The listing builds one solid part. Answer for the finished solid, in the listing's coordinates (mm). Coordinates: 2 decimals unless noted, no trailing zeros. Loops run counter-clockwise (first coordinate to the right, second up) from the corner with the lowest first, then second, coordinate; pieces in that order, holes last. Notation, with made-up numbers: (23, 55) - (65, 55) arc R14 ccw to (65, 82) - close; hole circle Ø9 at (2.25, 69). An arc over 180 degrees is marked (long way). Use one line per item in the form item = value. Start each with the question number.
```python
from build123d import *

# Parameters (mm, degrees)
SKETCH6_R                    = 29
SKETCH6_R_2                  = 20
INNER_RING_DEPTH             = 10
MOTOR_CONNECTOR_CUT_DEPTH    = 10
SKETCH9_R                    = 50
SKETCH9_R_2                  = 29
OUTSIDE_RING_EXTRUSION_DEPTH = 10
SKETCH12_R                   = 45
SKETCH12_R_2                 = 27.5
CUT_EXTRUDE6_DEPTH           = 55
SKETCH8_R                    = 2.987
MOTOR_CONNECTOR_HOLES_DEPTH  = 10
SKETCH10_R                   = 27.404299948
PATTERN_DEPTH                = 10
SKETCH13_R                   = 45
SKETCH13_R_2                 = 40
BOSS_EXTRUDE1_DEPTH          = 10


with BuildPart() as part:
    # Sketch6 → Inner Ring (new body)
    with BuildSketch(Plane.XY):
        Circle(SKETCH6_R)
        Circle(SKETCH6_R_2, mode=Mode.SUBTRACT)
    extrude(amount=-INNER_RING_DEPTH)

    # Sketch7 → Motor Connector Cut (add)
    with BuildSketch(Plane.XY):
        with BuildLine():
            ThreePointArc((20, 0), (19.840593925, 2.52008585), (19.364916731, 5))
            Line((19.364916731, 5), (9.999996731, 5))
            Line((9.999996731, 5), (9.999996731, -5))
            Line((9.999996731, -5), (19.364916731, -5))
            ThreePointArc((19.364916731, -5), (19.840593925, -2.52008585), (20, 0))
        make_face()
        with BuildLine():
            ThreePointArc((5, 19.364916731), (0, 20), (-5, 19.364916731))
            Line((-5, 19.364916731), (-5, 9.999996731))
            Line((-5, 9.999996731), (5, 9.999996731))
            Line((5, 9.999996731), (5, 19.364916731))
        make_face()
        with BuildLine():
            Line((-9.999996731, -5), (-9.999996731, 5))
            Line((-9.999996731, 5), (-19.364916731, 5))
            ThreePointArc((-19.364916731, 5), (-20, 0), (-19.364916731, -5))
            Line((-19.364916731, -5), (-9.999996731, -5))
        make_face()
        with BuildLine():
            Line((-5, -9.999996731), (-5, -19.364916731))
            ThreePointArc((-5, -19.364916731), (0, -20), (5, -19.364916731))
            Line((5, -19.364916731), (5, -9.999996731))
            Line((5, -9.999996731), (-5, -9.999996731))
        make_face()
    extrude(amount=-MOTOR_CONNECTOR_CUT_DEPTH)

    # Sketch9 → Outside Ring Extrusion (add)
    with BuildSketch(Plane.XY):
        Circle(SKETCH9_R)
        Circle(SKETCH9_R_2, mode=Mode.SUBTRACT)
    extrude(amount=-OUTSIDE_RING_EXTRUSION_DEPTH)

    # Sketch12 → Cut-Extrude6 (cut)
    with BuildSketch(Plane.XY):
        Circle(SKETCH12_R)
        Circle(SKETCH12_R_2, mode=Mode.SUBTRACT)
    extrude(amount=-CUT_EXTRUDE6_DEPTH, mode=Mode.SUBTRACT)

    # Sketch8 → Motor Connector Holes (cut)
    with BuildSketch(Plane.XY):
        with Locations((0, 17.75)):
            Circle(SKETCH8_R)
        with Locations((17.75, 0)):
            Circle(SKETCH8_R)
        with Locations((0, -17.75)):
            Circle(SKETCH8_R)
        with Locations((-17.75, 0)):
            Circle(SKETCH8_R)
    extrude(amount=-MOTOR_CONNECTOR_HOLES_DEPTH, mode=Mode.SUBTRACT)

    # Sketch10 → Pattern (add)
    with BuildSketch(Plane.XY):
        with BuildLine():
            ThreePointArc((24.317625284, 15.800414568), (34.856582319, 15.291767932), (43.817916626, 9.721954269))
            ThreePointArc((43.817916626, 9.721954269), (41.607188912, 16.793289988), (38.263814419, 23.404867172))
            ThreePointArc((38.263814419, 23.404867172), (32.064348025, 25.470287935), (25.530148518, 25.530148518))
            ThreePointArc((25.530148518, 25.530148518), (25.475284033, 32.034279432), (23.432821057, 38.209639668))
            ThreePointArc((23.432821057, 38.209639668), (20.212556871, 40.002288656), (16.856128399, 41.524812789))
            ThreePointArc((16.856128399, 41.524812789), (13.384732217, 42.767397097), (9.823095744, 43.720997037))
            ThreePointArc((9.823095744, 43.720997037), (15.312499865, 34.789679765), (15.800414568, 24.317625284))
            ThreePointArc((15.800414568, 24.317625284), (0, 29), (-15.800414568, 24.317625284))
            ThreePointArc((-15.800414568, 24.317625284), (-15.312499865, 34.789679765), (-9.823095744, 43.720997037))
            ThreePointArc((-9.823095744, 43.720997037), (-16.854754984, 41.52536899), (-23.432821057, 38.209639668))
            ThreePointArc((-23.432821057, 38.209639668), (-25.475284033, 32.034279432), (-25.530148518, 25.530148518))
            ThreePointArc((-25.530148518, 25.530148518), (-32.064348025, 25.470287935), (-38.263814419, 23.404867172))
            ThreePointArc((-38.263814419, 23.404867172), (-41.607188912, 16.793289988), (-43.817916626, 9.721954269))
            ThreePointArc((-43.817916626, 9.721954269), (-34.856582319, 15.291767932), (-24.317625284, 15.800414568))
            ThreePointArc((-24.317625284, 15.800414568), (-29, 0), (-24.317625284, -15.800414568))
            ThreePointArc((-24.317625284, -15.800414568), (-34.894848495, -15.279799844), (-43.87309253, -9.663767027))
            ThreePointArc((-43.87309253, -9.663767027), (-41.716263612, -16.713446711), (-38.435015504, -23.315212041))
            ThreePointArc((-38.435015504, -23.315212041), (-32.159621016, -25.454161245), (-25.530148518, -25.530148518))
            ThreePointArc((-25.530148518, -25.530148518), (-25.448803812, -32.190695038), (-23.285614603, -38.490703716))
            ThreePointArc((-23.285614603, -38.490703716), (-16.649731385, -41.799208281), (-9.559859326, -43.970581744))
            ThreePointArc((-9.559859326, -43.970581744), (-15.258354287, -34.962784804), (-15.800414568, -24.317625284))
            ThreePointArc((-15.800414568, -24.317625284), (0, -29), (15.800414568, -24.317625284))
            ThreePointArc((15.800414568, -24.317625284), (15.258354287, -34.962784804), (9.559859326, -43.970581744))
            ThreePointArc((9.559859326, -43.970581744), (16.649731385, -41.799208281), (23.285614603, -38.490703716))
            ThreePointArc((23.285614603, -38.490703716), (25.448803812, -32.190695038), (25.530148518, -25.530148518))
            ThreePointArc((25.530148518, -25.530148518), (32.159621016, -25.454161245), (38.435015504, -23.315212041))
            ThreePointArc((38.435015504, -23.315212041), (41.716263612, -16.713446711), (43.87309253, -9.663767027))
            ThreePointArc((43.87309253, -9.663767027), (34.894848495, -15.279799844), (24.317625284, -15.800414568))
            ThreePointArc((24.317625284, -15.800414568), (29, 0), (24.317625284, 15.800414568))
        make_face()
        with Locations((-0.095700052, 0)):
            Circle(SKETCH10_R, mode=Mode.SUBTRACT)
    extrude(amount=-PATTERN_DEPTH)

    # Sketch13 → Boss-Extrude1 (add)
    with BuildSketch(Plane(origin=(0, 0, -10), x_dir=(-1, 0, 0), z_dir=(0, 0, -1))):
        Circle(SKETCH13_R)
        Circle(SKETCH13_R_2, mode=Mode.SUBTRACT)
    extrude(amount=-BOSS_EXTRUDE1_DEPTH)


solid = part.part
```
(1) Each of these flat-tipped pins is pushed along its axis until it touches: pin 1 Ø5.5 at (x, y) = (0, 17.75) entering from -Z; pin 2 Ø8 at (x, y) = (0, -17.75) entering from -Z; pin 3 Ø1 at (y, z) = (21.5, -4.5) entering from -X; pin 4 Ø3 at (y, z) = (-2, -4.5) entering from +X. Where does it stop, or does it pass through?
(2) A cutting plane is placed at A-A (y = 0). Determine the outline of the cut face in (x, z).
(3) Find the intervals of material crossed by probe 1 along Y at (x, z) = (0, -2.75); probe 2 along X at (y, z) = (-12, -7.5); probe 3 along X at (y, z) = (13, -5.5), in increasing order. Write a range as from..to.
(4) A cutting plane is placed at D-D (z = -5). State how many separate pieces and enclosed holes the cut face has, then the cut area to 3 significant figures.
(5) Determine the mould class of faces 1 (the face through (14.766, 0.131, -4.93)), 2 (the face through (29, 0, -5)) for opening direction X: +X half, -X half, draft (parallel to the pull), parting line (faces both ways), or undercut.
(6) A cutting plane is placed at C-C (y = -17.75). Determine the outline of the cut face in (x, z), then the cut area to 3 significant figures.
(7) A cutting plane is placed at B-B (x = -7). Determine the outline of the cut face in (y, z) (1 decimal).
Evaluation:
q1.pin_1 = through
q1.pin_2 = -10
q1.pin_3 = -45.38
q1.pin_4 = 50
q2.outline = (-50, -10) - (-40, -10) - (-40, 0) - (-50, 0) - close; (-29, -10) - (-20.74, -10) - (-20.74, 0) - (-29, 0) - close; (-14.76, -10) - (-10, -10) - (-10, 0) - (-14.76, 0) - close; (10, -10) - (14.76, -10) - (14.76, 0) - (10, 0) - close; (20.74, -10) - (29, -10) - (29, 0) - (20.74, 0) - close; (40, -10) - (50, -10) - (50, 0) - (40, 0) - close
q3.probe_1 = -50..-40, -29..-20.74, -14.76..-10, 10..14.76, 20.74..29, 40..50
q3.probe_2 = -48.54..-38.16, -26.4..-16, -5..5, 16..26.4, 38.16..48.54
q3.probe_3 = -48.28..-37.83, -25.92..-15.2, -5..5, 15.2..25.92, 37.83..48.28
q4.separate_pieces = 1
q4.enclosed_holes = 13
q4.area = 5,380 mm^2
q5.face_1 = undercut
q5.face_2 = undercut
q6.outline = (-46.74, -10) - (-9.22, -10) - (-9.22, 0) - (-46.74, 0) - close; (-5, -10) - (-2.99, -10) - (-2.99, 0) - (-5, 0) - close; (2.99, -10) - (5, -10) - (5, 0) - (2.99, 0) - close; (9.22, -10) - (46.74, -10) - (46.74, 0) - (9.22, 0) - close
q6.area = 791 mm^2
q7.outline = (-49.5, -10) - (-39.4, -10) - (-39.4, 0) - (-49.5, 0) - close; (-28.1, -10) - (-18.7, -10) - (-18.7, 0) - (-28.1, 0) - close; (18.7, -10) - (28.1, -10) - (28.1, 0) - (18.7, 0) - close; (39.4, -10) - (49.5, -10) - (49.5, 0) - (39.4, 0) - close
